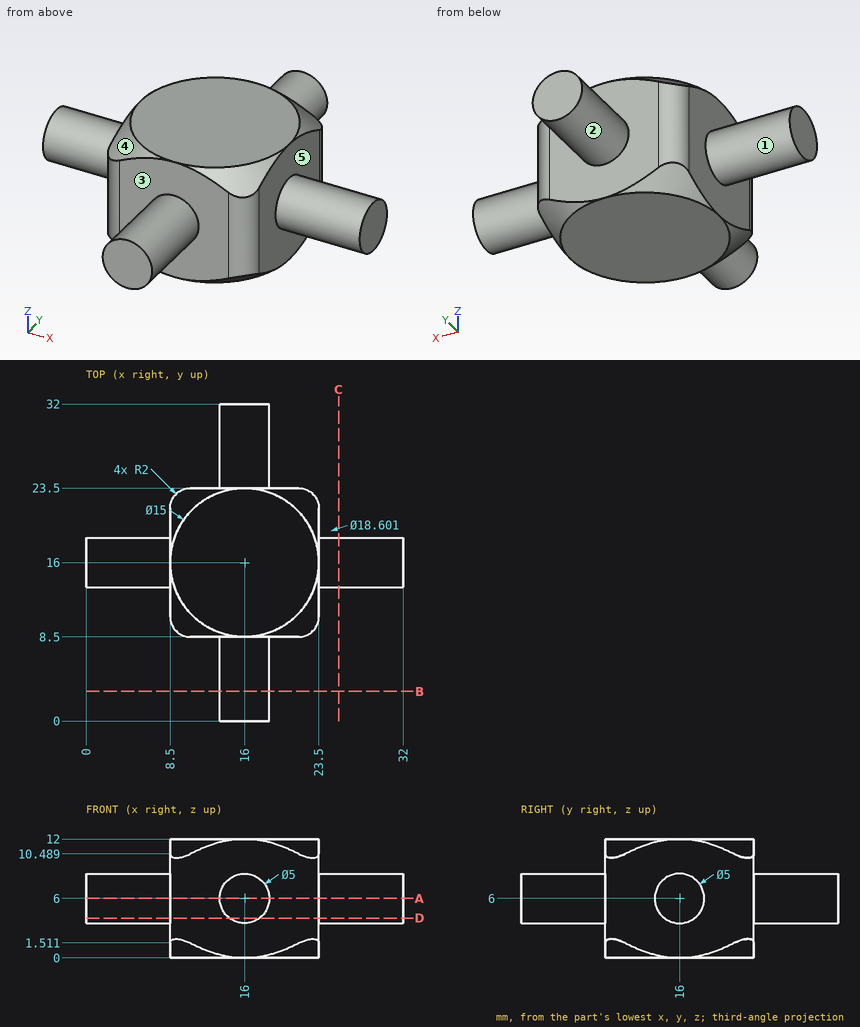
Print and shaded views of the part. All mm, measured from the part's lowest x, y and z. A direction names the side the tool comes from. Coordinates: 2 decimals unless noted, no trailing zeros. Order: outer loops, then holes, each group sorted by start corner. A loop starts at its lowest first (then second) coordinate and runs counter-clockwise, first axis right, second up. Notation, with made-up numbers: (84.25, 76) -> (141.25, 76) arc R23 cw to (141.25, 114) -> close; hole circle Ø2 at (66, -36.75). An arc over 180 degrees is marked (long way). Answer as a JSON object with one key per item and string values. Group by question number.
1) Cut at A-A, the plane z = 6. Write the cut outline in (x, y).
2) Flat gauge pins, fed straight in: pin 1 (1.5 mm diameter, centred on y = 24, z = 2, fed in from -X); pin 2 (4 mm diameter, centred on x = 12, z = 3.5, fed in from +Y); pin 3 (4 mm diameter, centred on y = 19.5, z = 7, fed in from +X). Where does each tip first touch, or does it go through?
3) Cut at B-B, the plane y = 3. Write the cut outline in (x, z), then the cut area to 3 significant figures.
4) Drill centre lines: L1, parallel to X at y = 21, z = 9; L2, parallel to X at y = 22, z = 5.5. Where is each one in solid material? Low to high.
5) Cut at D-D, the plane z = 4. Write the cut outline in (x, y).
6) Which spindle directions (+Z, -Z, +X, -X, +Y, -Y) get a long thin tool onto all of the face, cutting with end or side? Do the marked faces 1, 2, 3, 4 and 5. Say none if no direction does.
Check values:
{
 "1": {"outline": "(0, 13.5) -> (8.5, 13.5) -> (8.5, 10.5) arc R2 ccw to (10.5, 8.5) -> (13.5, 8.5) -> (13.5, 0) -> (18.5, 0) -> (18.5, 8.5) -> (21.5, 8.5) arc R2 ccw to (23.5, 10.5) -> (23.5, 13.5) -> (32, 13.5) -> (32, 18.5) -> (23.5, 18.5) -> (23.5, 21.5) arc R2 ccw to (21.5, 23.5) -> (18.5, 23.5) -> (18.5, 32) -> (13.5, 32) -> (13.5, 23.5) -> (10.5, 23.5) arc R2 ccw to (8.5, 21.5) -> (8.5, 18.5) -> (0, 18.5) -> close"},
 "2": {"pin 1": "stops at x = 9.53", "pin 2": "stops at y = 23.5", "pin 3": "stops at x = 32"},
 "3": {"outline": "circle Ø5 at (16, 6)", "area": "19.6 mm²"},
 "4": {"L1": "x = 8.5 to 23.5", "L2": "x = 8.56 to 23.44"},
 "5": {"outline": "(0, 14.5) -> (8.5, 14.5) -> (8.5, 10.5) arc R2 ccw to (10.5, 8.5) -> (14.5, 8.5) -> (14.5, 0) -> (17.5, 0) -> (17.5, 8.5) -> (21.5, 8.5) arc R2 ccw to (23.5, 10.5) -> (23.5, 14.5) -> (32, 14.5) -> (32, 17.5) -> (23.5, 17.5) -> (23.5, 21.5) arc R2 ccw to (21.5, 23.5) -> (17.5, 23.5) -> (17.5, 32) -> (14.5, 32) -> (14.5, 23.5) -> (10.5, 23.5) arc R2 ccw to (8.5, 21.5) -> (8.5, 17.5) -> (0, 17.5) -> close"},
 "6": {"face 1": "-X", "face 2": "+Y", "face 3": "-Y", "face 4": "+Z, -X, -Y", "face 5": "+X"}
}
